from build123d import *

# Parameters (mm, degrees)
F0_W     = 101.6
F0_H     = 12.7
F1_DEPTH = 25.4
F2_W     = 168.6520413041
F2_H     = 61.9295807295
F2_H_2   = 759.2988385411
F3_DEPTH = 25.401


with BuildPart() as f1:
    # F0 (on Front) → F1 (new body)
    with BuildSketch(Plane.XZ):
        Polygon((128.9281710505, -699.8807162309), (128.9281710505, 183.2772837691), (-93.3218289495, 183.2772837691), (-93.3218289495, 107.0772837691), (-106.0218289495, 107.0772837691), (-106.0218289495, 30.8772837691), (-93.3218289495, 30.8772837691), (-93.3218289495, -45.3227162309), (-106.0218289495, -45.3227162309), (-106.0218289495, -121.5227162309), (-93.3218289495, -121.5227162309), (-93.3218289495, -197.7227162309), (-106.0218289495, -197.7227162309), (-106.0218289495, -273.9227162309), (-93.3218289495, -273.9227162309), (-93.3218289495, -350.1227162309), (-106.0218289495, -350.1227162309), (-106.0218289495, -426.3227162309), (-93.3218289495, -426.3227162309), (-93.3218289495, -502.5227162309), (-106.0218289495, -502.5227162309), (-106.0218289495, -578.7227162309), (-93.3218289495, -578.7227162309), (-93.3218289495, -699.8807162309), (8.2781710505, -699.8807162309), align=None)
        Polygon((351.1781710505, 183.2772837691), (128.9281710505, 183.2772837691), (128.9281710505, -699.8807162309), (249.5781710505, -699.8807162309), (351.1781710505, -699.8807162309), (351.1781710505, -578.7227162309), (363.8781710505, -578.7227162309), (363.8781710505, -502.5227162309), (351.1781710505, -502.5227162309), (351.1781710505, -426.3227162309), (363.8781710505, -426.3227162309), (363.8781710505, -350.1227162309), (351.1781710505, -350.1227162309), (351.1781710505, -273.9227162309), (363.8781710505, -273.9227162309), (363.8781710505, -197.7227162309), (351.1781710505, -197.7227162309), (351.1781710505, -121.5227162309), (363.8781710505, -121.5227162309), (363.8781710505, -45.3227162309), (351.1781710505, -45.3227162309), (351.1781710505, 30.8772837691), (363.8781710505, 30.8772837691), (363.8781710505, 107.0772837691), (351.1781710505, 107.0772837691), align=None)
        with Locations((-42.5218289495, -706.2307162309)):
            Rectangle(F0_W, F0_H)
        with Locations((300.3781710505, -706.2307162309)):
            Rectangle(F0_W, F0_H)
    extrude(amount=F1_DEPTH)

    # F2 (on face) → F3 (cut, through all)
    with BuildSketch(Plane.XZ.offset(25.4)):
        with Locations((213.2541917026, 152.3124934044)):
            Rectangle(F2_W, F2_H)
        with Locations((44.6021503985, 152.3124934044)):
            Rectangle(F2_W, F2_H)
        with Locations((213.2541917026, -258.3017162309)):
            Rectangle(F2_W, F2_H_2)
        with Locations((44.6021503985, -258.3017162309)):
            Rectangle(F2_W, F2_H_2)
    extrude(amount=-F3_DEPTH, mode=Mode.SUBTRACT)


solid = f1.part
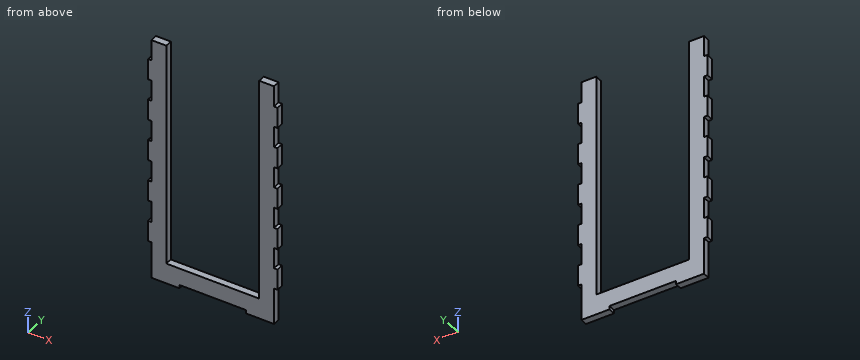
Here's how the part is built. I have some questions about the finished solid (model axes, mm). Coordinates: 2 decimals unless noted, no trailing zeros. Write each loop counter-clockwise with the first axis right and the second up, starting at its lowest first coordinate (ties: lowest second). Pieces come first, ordered by that corner, then holes.
Item 1: I want a section at C-C on x = -2.5. Write out the boundary of the cut face in (y, z), and give its area (3 significant figures).
Item 2: I want a section at B-B on z = -486. Write out the boundary of the cut face in (x, y), and give its area (3 significant figures).
Item 3: I want a section at A-A on z = -221. Write out the boundary of the cut face in (x, y).
Item 4: If I drill on line 1 (X direction, y = -23, z = -323); line 2 (X direction, y = -7.75, z = -255); line 3 (Z direction, x = 200.5, y = -12), over which ranges is the centre line in solid material (lowest first)?
Item 5: I want a section at D-D on x = 201.5. Write out the boundary of the cut face in (y, z), and give its area (3 significant figures).
Item 6: Will these pins go through, and if not, where does the flat tip stop? pin 1 (8 mm diameter, centred on y = -16, z = -484, fed in from -X); pin 2 (4 mm diameter, centred on x = -100, y = -8.5, fed in from -Z); pin 3 (12.5 mm diameter, centred on y = -7.5, z = -171.5, fed in from +X).
Findings below:
1. outline: (-25.4, -712.58) - (0, -712.58) - (0, -637.95) - (-25.4, -637.95) - close
1. area: 1,900 mm2
2. outline: (-93.32, -25.4) - (-39.72, -25.4) - (-39.72, 0) - (-93.32, 0) - close; (297.58, -25.4) - (351.18, -25.4) - (351.18, 0) - (297.58, 0) - close
2. area: 2,720 mm2
3. outline: (-106.02, -25.4) - (-39.72, -25.4) - (-39.72, 0) - (-106.02, 0) - close; (297.58, -25.4) - (363.88, -25.4) - (363.88, 0) - (297.58, 0) - close
4. line 1: x = -93.32 to -39.72, 297.58 to 351.18
4. line 2: x = -106.02 to -39.72, 297.58 to 363.88
4. line 3: z = -699.88 to -637.95
5. outline: (-25.4, -699.88) - (0, -699.88) - (0, -637.95) - (-25.4, -637.95) - close
5. area: 1,570 mm2
6. pin 1: stops at x = -93.32
6. pin 2: stops at z = -578.72
6. pin 3: stops at x = 351.18
